Answer from the drawing. Dimensions are ordinates in mm from the lowest x, y and z of the part. A direction names the side the tool comes from. Coordinates: 2 decimals unless noted, no trailing zeros. Order: outer loops, then holes, each group sorted by start corner. A loop starts at its lowest first (then second) coordinate and runs counter-clockwise, first axis right, second up. Notation, with made-up numbers: (76.25, 32) -> (94.25, 32) arc R27 ccw to (94.25, 54) -> close; hole circle Ø10 at (80.5, 28.5). An arc over 180 degrees is marked (long way). Answer in a Markdown table with one row per item.
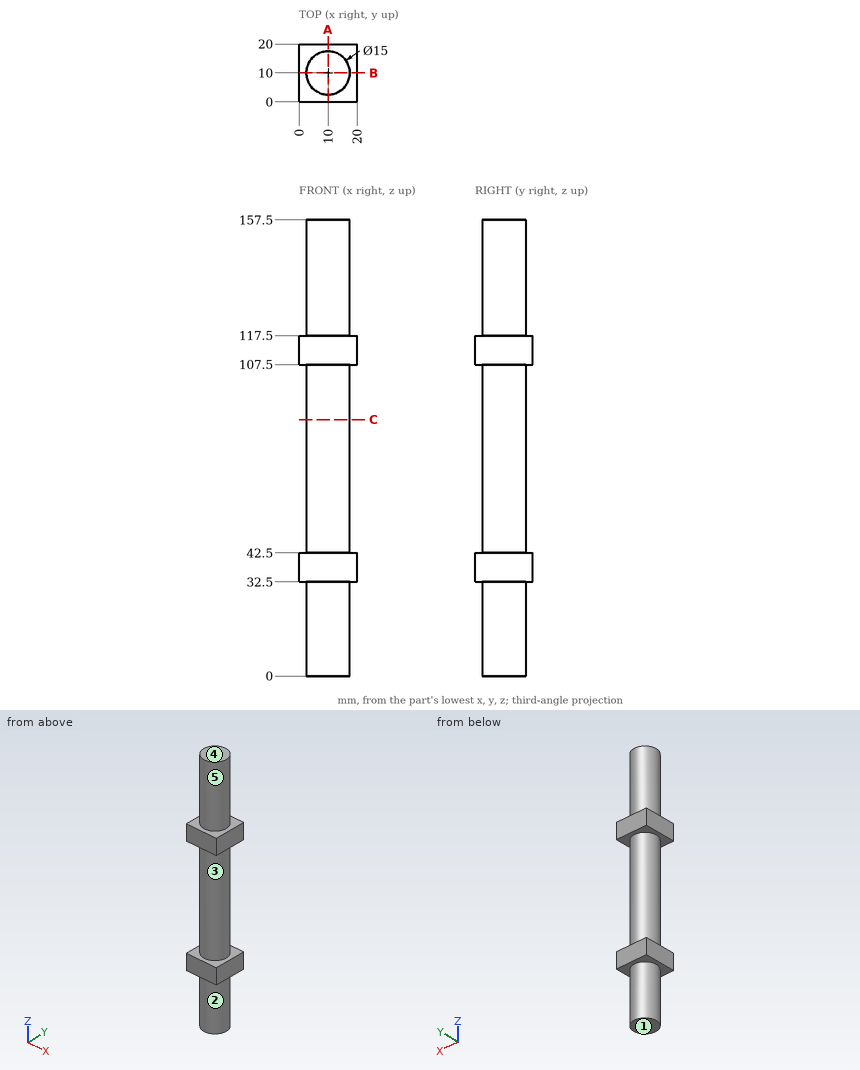
(1) Which of the six approach directions +Z, -Z, +X, -X, +Y, -Y give full straight-line access (tool end or side, diameter ignored) to the marked faces 1 and 2?
Check values:
| item | result |
|---|---|
| face 1 | -Z, +X, -X, +Y, -Y |
| face 2 | -Z |
(2) A cutting plane is placed at C-C, the plane z = 88.5. Determine the outline of the cut face in (x, y).
Check values:
| item | result |
|---|---|
| outline | circle Ø15 at (10, 10) |
(3) For a pull along Z with two mould halves and no side action, classify the marked faces 3, 4 and 5 as released by +Z, released by -Z, zero draft, split by the parting line, or undercut.
Check values:
| item | result |
|---|---|
| face 3 | undercut |
| face 4 | released by +Z |
| face 5 | zero draft |
(4) Find the intervals of material crossed by line 1 along Z through (x, y) = (2, 16.5); line 2 along Y through (x, z) = (9.75, 106.5), in increasing order. Write a range as from..to.
Check values:
| item | result |
|---|---|
| line 1 | 32.5..42.5, 107.5..117.5 |
| line 2 | 2.5..17.5 |
(5) A cutting plane is placed at A-A, the plane x = 10. Determine the outline of the cut face in (y, z).
Check values:
| item | result |
|---|---|
| outline | (0, 32.5) -> (2.5, 32.5) -> (2.5, 0) -> (17.5, 0) -> (17.5, 32.5) -> (20, 32.5) -> (20, 42.5) -> (17.5, 42.5) -> (17.5, 107.5) -> (20, 107.5) -> (20, 117.5) -> (17.5, 117.5) -> (17.5, 157.5) -> (2.5, 157.5) -> (2.5, 117.5) -> (0, 117.5) -> (0, 107.5) -> (2.5, 107.5) -> (2.5, 42.5) -> (0, 42.5) -> close |
(6) Flat-ended cylindrical pins translate along their axes: pin 1 (12 mm diameter, centred on x = 9.5, z = 24.5, fed in from -Y); pin 2 (1 mm diameter, centred on y = 8, z = 27.5, fed in from +X); pin 3 (3 mm diameter, centred on x = 3, z = 76, fed in from +Y). Find the tip coordinate at first contact, or state that the pin passes through.
Check values:
| item | result |
|---|---|
| pin 1 | y = 2.5 |
| pin 2 | x = 17.35 |
| pin 3 | y = 15.1 |
